from build123d import *

# Parameters (mm, degrees)
SKETCH1_R                 = 19
BOSS_EXTRUDE1_DEPTH       = 35
BOSS_EXTRUDE2_START       = 35
SKETCH2_R                 = 10
BOSS_EXTRUDE2_DEPTH       = 5
BOSS_EXTRUDE3_START       = 40
SKETCH3_R                 = 3
BOSS_EXTRUDE3_DEPTH       = 13
CUT_EXTRUDE1_START        = -10
CUT_EXTRUDE1_DEPTH        = 10
M3X0_5_TAPPED_HOLE1_D     = 2.5
M3X0_5_TAPPED_HOLE1_DEPTH = 7.5
M3X0_5_TAPPED_HOLE1_TIP   = 0.751075774


with BuildPart() as part:
    # Sketch1 → Boss-Extrude1 (new body)
    with BuildSketch(Plane.XY):
        Circle(SKETCH1_R)
    extrude(amount=BOSS_EXTRUDE1_DEPTH)

    # Sketch2 → Boss-Extrude2 (add)
    with BuildSketch(Plane.XY.offset(BOSS_EXTRUDE2_START)):
        Circle(SKETCH2_R)
    extrude(amount=BOSS_EXTRUDE2_DEPTH)

    # Sketch3 → Boss-Extrude3 (add)
    with BuildSketch(Plane.XY.offset(BOSS_EXTRUDE3_START)):
        with Locations(Location((0, 0, 0), (0, 0, 180))):
            Circle(SKETCH3_R)
    extrude(amount=BOSS_EXTRUDE3_DEPTH)

    # Sketch4 → Cut-Extrude1 (cut)
    with BuildSketch(Plane.XY.offset(53).offset(CUT_EXTRUDE1_START)):
        with BuildLine():
            Line((-1.658312395, 2.5), (1.658312395, 2.5))
            ThreePointArc((1.658312395, 2.5), (0, 3), (-1.658312395, 2.5))
        make_face()
    extrude(amount=CUT_EXTRUDE1_DEPTH, mode=Mode.SUBTRACT)

    # M3x0.5 Tapped Hole1
    with Locations(Plane.XY.offset(35)):
        with Locations((0, 14), (7.5, 12.990381057), (12.124355653, -7), (7.5, -12.990381057), (-12.124355653, -7), (-15, 0)):
            Hole(M3X0_5_TAPPED_HOLE1_D / 2, depth=M3X0_5_TAPPED_HOLE1_DEPTH)
            with Locations((0, 0, -(M3X0_5_TAPPED_HOLE1_DEPTH + M3X0_5_TAPPED_HOLE1_TIP / 2))):  # 118° drill point
                Cone(0, M3X0_5_TAPPED_HOLE1_D / 2, M3X0_5_TAPPED_HOLE1_TIP, mode=Mode.SUBTRACT)


solid = part.part
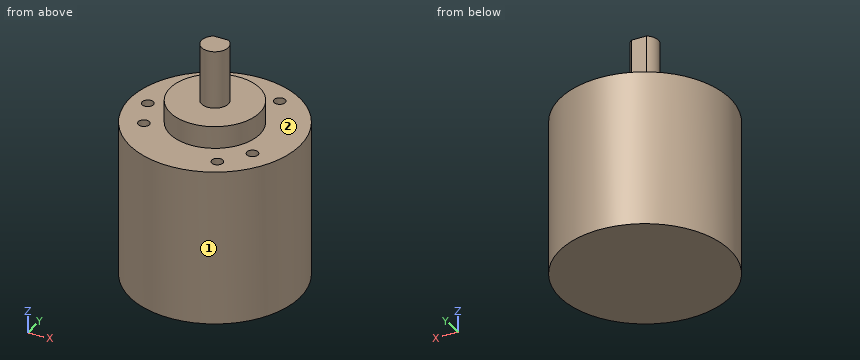
Verification items for the finished model (mm, model axes). Face numbers are marked on the shaded views. A direction names the side the tool comes from. Give positions to 0.01 mm unless a question says otherwise; leave off trailing zeros. Order: outer loops, then holes, each group sorted by start corner. A loop starts at its lowest first (then second) coordinate and runs counter-clockwise, first axis right, second up. Notation, with made-up numbers: (18.5, -32) -> (58.5, -32) arc R28 ccw to (58.5, 5) -> close; hole circle Ø7 at (77, -5). An arc over 180 degrees is marked (long way). Answer as CSV lines item,"result".
Q1. Access from +Z, -Z, +X, -X, +Y, -Y to the whole of each face (thin tool, end or side, straight path). Record for the marked faces 1 and 2.
Solutions:
face 1,"+Z, -Z"
face 2,"+Z"
Q2. Sectioned sample at A-A on z = 36. Record the cut outline in (x, y).
Solutions:
outline,"circle Ø20 at (0, 0)"
Q3. Sectioned sample at B-B on x = -9. Record the cut outline in (y, z), plus the area to 3 significant figures.
Solutions:
outline,"(-16.73, 0) -> (16.73, 0) -> (16.73, 35) -> (4.36, 35) -> (4.36, 40) -> (-4.36, 40) -> (-4.36, 35) -> (-16.73, 35) -> close"
area,"1,210 mm²"
Q4. Sectioned sample at D-D on z = 7.5. Record the cut outline in (x, y), plus the area to 3 significant figures.
Solutions:
outline,"circle Ø38 at (0, 0)"
area,"1,130 mm²"
Q5. Depth check by flat-ended pin: pin 1 (1 mm diameter, centred on y = 2, z = 27.5, fed in from -X); pin 2 (3 mm diameter, centred on x = 12.12, y = -7, fed in from -Z); pin 3 (10 mm diameter, centred on x = 0.5, z = 23.5, fed in from +Y); pin 4 (1.5 mm diameter, centred on x = -15, y = 0, fed in from +Z). Enter the tip coordinate at first touch or a pass-through.
Solutions:
pin 1,"stops at x = -18.94"
pin 2,"stops at z = 0"
pin 3,"stops at y = 19"
pin 4,"stops at z = 27.2"
Q6. Sectioned sample at C-C on y = 8.5. Record the cut outline in (x, z).
Solutions:
outline,"(-16.99, 0) -> (16.99, 0) -> (16.99, 35) -> (5.27, 35) -> (5.27, 40) -> (-5.27, 40) -> (-5.27, 35) -> (-16.99, 35) -> close"
Q7. Scan lines: probe 1 along Y at (x, z) = (0, 31); probe 2 along X at (y, z) = (14, 33.75); probe 3 along Y at (x, z) = (7, 31). Record each from-to range of solid material in increasing order.
Solutions:
probe 1,"y = -19 to 12.75, 15.25 to 19"
probe 2,"x = -12.85 to -1.25, 1.25 to 6.76, 8.24 to 12.85"
probe 3,"y = -17.66 to -14.14, -11.84 to 11.84, 14.14 to 17.66"
